from build123d import *
from build123d.topology import SkipClean

# Parameters (mm, degrees)
SKETCH2_W               = 14
SKETCH2_H               = 6
BOSS_EXTRUDE1_DEPTH     = 4
SKETCH3_W               = 4
SKETCH3_H               = 6
BOSS_EXTRUDE2_DEPTH     = 12
CUT_EXTRUDE1_DEPTH      = 22.470910554
CUT_EXTRUDE1_DEPTH_BACK = 22.470910554
SKETCH4_R               = 1.5
BOSS_EXTRUDE3_START     = 1
SKETCH5_R               = 2.5
SKETCH5_R_2             = 1.5
BOSS_EXTRUDE3_DEPTH     = 1
SKETCH6_R               = 2.5
SKETCH6_R_2             = 1.5
BOSS_EXTRUDE4_DEPTH     = 1
SKETCH7_W               = 11
SKETCH7_H               = 6
SKETCH7_R               = 1
BOSS_EXTRUDE5_DEPTH     = 4
FILLET1_R               = 2
FILLET2_R               = 3


with BuildPart() as part:
    # Sketch2 → Boss-Extrude1 (new body)
    with BuildSketch(Plane(origin=(0, 0, 0), x_dir=(1, 0, 0), z_dir=(0, 1, 0))):
        Rectangle(SKETCH2_W, SKETCH2_H)
    extrude(amount=BOSS_EXTRUDE1_DEPTH)

    # Sketch3 → Boss-Extrude2 (add)
    with BuildSketch(Plane(origin=(0, 4, 0), x_dir=(1, 0, 0), z_dir=(0, 1, 0))):
        with Locations((-5, 0)):
            Rectangle(SKETCH3_W, SKETCH3_H)
        with Locations((5, 0)):
            Rectangle(SKETCH3_W, SKETCH3_H)
    extrude(amount=BOSS_EXTRUDE2_DEPTH)

    # Sketch4 → Cut-Extrude1 (cut, two sides: drawn at the far end of the back side and taken through both)
    with BuildSketch(Plane(origin=(7, 0, 0), x_dir=(0, 0, -1), z_dir=(1, 0, 0)).offset(-CUT_EXTRUDE1_DEPTH_BACK)):
        with Locations((0, 12)):
            Circle(SKETCH4_R)
    extrude(amount=CUT_EXTRUDE1_DEPTH + CUT_EXTRUDE1_DEPTH_BACK, mode=Mode.SUBTRACT)

    # Sketch5 → Boss-Extrude3 (add)
    with BuildSketch(Plane(origin=(-3, 0, 0), x_dir=(0, 0, -1), z_dir=(1, 0, 0)).offset(BOSS_EXTRUDE3_START)):
        with Locations(Location((0, 12, 0), (0, 0, 180))):
            Circle(SKETCH5_R)
        with Locations((0, 12)):
            Circle(SKETCH5_R_2, mode=Mode.SUBTRACT)
    extrude(amount=-BOSS_EXTRUDE3_DEPTH)

    # Sketch6 → Boss-Extrude4 (add)
    with SkipClean():  # the faces are left unmerged after this step: merging them gives an invalid solid
        with BuildSketch(Plane.ZY.offset(-3)):
            with Locations((0, 12)):
                Circle(SKETCH6_R)
            with Locations((0, 12)):
                Circle(SKETCH6_R_2, mode=Mode.SUBTRACT)
        extrude(amount=BOSS_EXTRUDE4_DEPTH)

    # Sketch7 → Boss-Extrude5 (add)
    # profile 1 of 2: a face of its own
    with SkipClean():  # the faces are left unmerged after this step: merging them gives an invalid solid
        with BuildSketch(Plane(origin=(0, 4, 0), x_dir=(1, 0, 0), z_dir=(0, 1, 0))):
            with Locations((12.5, 0)):
                Rectangle(SKETCH7_W, SKETCH7_H)
            with Locations(Location((15, 0, 0), (0, 0, 270))):
                Circle(SKETCH7_R, mode=Mode.SUBTRACT)
        # profile 2 of 2: a face of its own
        with BuildSketch(Plane(origin=(0, 4, 0), x_dir=(1, 0, 0), z_dir=(0, 1, 0))):
            with Locations((-12.5, 0)):
                Rectangle(SKETCH7_W, SKETCH7_H)
            with Locations(Location((-15, 0, 0), (0, 0, 270))):
                Circle(SKETCH7_R, mode=Mode.SUBTRACT)
        extrude(amount=-BOSS_EXTRUDE5_DEPTH)

    # Fillet1
    fillet1_edges = [part.edges().sort_by_distance(p)[0] for p in [
        (18, 2, -3),
        (18, 2, 3),
        (-18, 2, 3),
        (-18, 2, -3),
    ]]
    fillet(fillet1_edges, radius=FILLET1_R)

    # Fillet2
    fillet2_edges = [part.edges().sort_by_distance(p)[0] for p in [
        (-5, 16, -3),
        (5, 16, -3),
        (5, 16, 3),
        (-5, 16, 3),
    ]]
    fillet(fillet2_edges, radius=FILLET2_R - 0.0001)  # a hair under: the kernel refuses the full size


solid = part.part
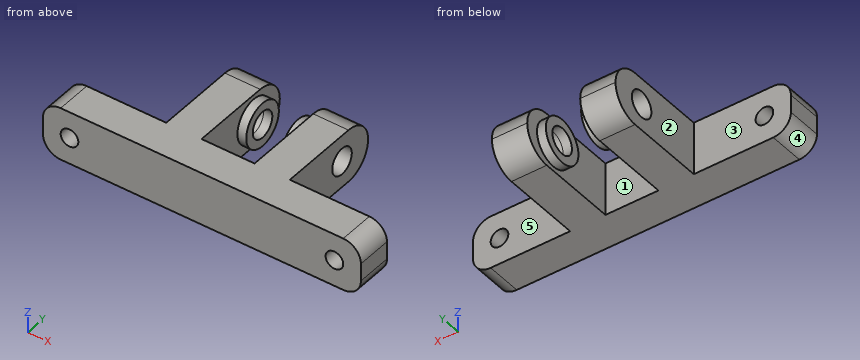
Source: CAD feature listing. Evaluate the final solid. Frame: model axes, mm. Face numbers are marked on the shaded views. A direction names the side the tool comes from. Round coordinates to 2 decimals unless told otherwise and drop trailing zeros. Loops run counter-clockwise (first coordinate to the right, second up) from the corner with the lowest first, then second, coordinate; pieces in that order, holes last. Notation, with made-up numbers: M 38,71.25 L 63,71.25 A36 cw 63,110.25 Z; hole C -9,8 d2. An arc over 180 degrees is marked long. Answer as CSV lines item,"result".
Q1. Contact query for flat-ended pins moving along their axis: pin 1 (3 mm diameter, centred on x = 15, z = 0, fed in from +Y); pin 2 (8 mm diameter, centred on x = -8, y = 11, fed in from +Z); pin 3 (1.8 mm diameter, centred on y = 7.5, z = 1, fed in from +X). Output: stop coordinate, or through.
Verdict:
pin 1,"stops at y = 4"
pin 2,"stops at z = 3"
pin 3,"stops at x = 7"
Q2. Cut plane B-B (y = 4.5). Return the cut outline in (x, z).
Verdict:
outline,"M -7,-3 L -3,-3 L -3,3 L -7,3 Z; M 3,-3 L 7,-3 L 7,3 L 3,3 Z"
Q3. Line query: line 1 along Y through (x, z) = (4.25, 0); line 2 along X through (y, z) = (14.5, -1.5); line 3 along X through (y, z) = (2, -0.25). Output: solid intervals per line, ascending.
Verdict:
line 1,"y = 0 to 10.5, 13.5 to 16"
line 2,"x = -7 to -3, 3 to 7"
line 3,"x = -18 to -15.97, -14.03 to 14.03, 15.97 to 18"
Q4. Cut plane A-A (y = 12). Return the cut outline in (x, z).
Verdict:
outline,"M -7,-3 L -3,-3 L -3,-2.5 L -2,-2.5 L -2,-1.5 L -7,-1.5 Z; M -7,1.5 L -2,1.5 L -2,2.5 L -3,2.5 L -3,3 L -7,3 Z; M 2,-2.5 L 3,-2.5 L 3,-3 L 7,-3 L 7,-1.5 L 2,-1.5 Z; M 2,1.5 L 7,1.5 L 7,3 L 3,3 L 3,2.5 L 2,2.5 Z"
Q5. Cut plane C-C (x = -15). Return the cut outline in (y, z), plus the area to 3 significant figures.
Verdict:
outline,"M 0,-3 L 4,-3 L 4,-1 L 0,-1 Z; M 0,1 L 4,1 L 4,3 L 0,3 Z"
area,"16.0 mm^2"
Q6. Reachability of the marked faces 4 and 5 from +Z, -Z, +X, -X, +Y, -Y: full face, straight path, thin tool, end or side. Return the list, or none.
Verdict:
face 4,"-Z, -X, +Y, -Y"
face 5,"+Z, -Z, +X, +Y"
Q7. Pull-direction query (X, two-part tool) for the marked faces 1, 2 and 3; classes: +X half, -X half, draft (parallel to the pull), parting line (faces both ways), or undercut.
Verdict:
face 1,"undercut"
face 2,"-X half"
face 3,"draft"
